Design review of the part built by this model. Coordinates are the model's own, in mm. Give positions to 0.01 mm unless a question says otherwise; leave off trailing zeros. Write each loop counter-clockwise with the first axis right and the second up, starting at its lowest first coordinate (ties: lowest second). Pieces come first, ordered by that corner, then holes. Notation, with made-up numbers: M 45.25,7 L 81.25,7 A13 cw 81.25,23 Z; hole C -15.5,-26 d5. An arc over 180 degrees is marked long. Use one line per item in the form item = value. Start each with the question number.
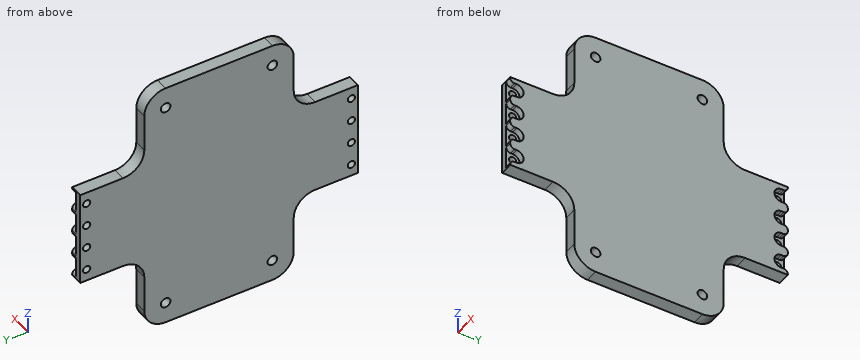
from build123d import *

# Parameters (mm, degrees)
SKETCH_1_W                  = 6
SKETCH_1_H                  = 30
EXTRUDE_1_DEPTH             = 130
EXTRUDE_3_DEPTH             = 6
HOLE_WIZARD_M31_D           = 3.4
HOLE_WIZARD_M31_CBORE_D     = 6.5
HOLE_WIZARD_M31_CBORE_DEPTH = 3
HOLE_WIZARD_M41_D           = 4.5
FILLET_1_R                  = 10
SKETCH_17_W                 = 6.5
SKETCH_17_H                 = 5
CUT_EXTRUDE_1_DEPTH         = 3
FILLET_2_R                  = 2


with BuildPart() as part:
    # Эскиз1 → Бобышка-Вытянуть1 (new body)
    with BuildSketch(Plane(origin=(0, 0, 0), x_dir=(1, 0, 0), z_dir=(0, 1, 0))):
        with Locations((3, -15)):
            Rectangle(SKETCH_1_W, SKETCH_1_H)
    extrude(amount=EXTRUDE_1_DEPTH)

    # Эскиз11 → Бобышка-Вытянуть3 (add)
    with BuildSketch(Plane(origin=(6, 0, 0), x_dir=(0, 0, -1), z_dir=(1, 0, 0))):
        Polygon((-37.5, 124), (-37.5, 100), (-75, 100), (-75, 30), (-37.5, 30), (-37.5, 6), (-37.5, 0), (7.5, 0), (7.5, 6), (7.5, 30), (45, 30), (45, 100), (7.5, 100), (7.5, 124), (7.5, 130), (-37.5, 130), align=None)
    extrude(amount=-EXTRUDE_3_DEPTH)

    # Цековка для винта с внутренним шестигранником M31 (through all)
    with Locations(Plane(origin=(6, 0, 0), x_dir=(0, 0, -1), z_dir=(1, 0, 0))):
        with Locations((-31.875, 127), (-20.625, 127), (-9.375, 127), (1.875, 127), (-31.875, 3), (-20.625, 3), (-9.375, 3), (1.875, 3)):
            CounterBoreHole(HOLE_WIZARD_M31_D / 2, HOLE_WIZARD_M31_CBORE_D / 2, HOLE_WIZARD_M31_CBORE_DEPTH)

    # Отверстие с зазором M41 (through all)
    with Locations(Plane(origin=(6, 0, 0), x_dir=(0, 0, -1), z_dir=(1, 0, 0))):
        with Locations((-65, 90), (-65, 40), (35, 40), (35, 90)):
            Hole(HOLE_WIZARD_M41_D / 2)

    # Скругление1
    fillet_1_edges = [part.edges().sort_by_distance(p)[0] for p in [
        (3, 100, -7.5),
        (3, 100, -45),
        (3, 30, -45),
        (3, 30, -7.5),
        (3, 30, 37.5),
        (3, 30, 75),
        (3, 100, 75),
        (3, 100, 37.5),
    ]]
    fillet(fillet_1_edges, radius=FILLET_1_R)

    # Эскиз17 → Вырез-Вытянуть1 (cut)
    with BuildSketch(Plane(origin=(6, 0, 0), x_dir=(0, 0, -1), z_dir=(1, 0, 0))):
        with Locations((-9.375, 129.5)):
            Rectangle(SKETCH_17_W, SKETCH_17_H)
        with Locations((1.875, 129.5)):
            Rectangle(SKETCH_17_W, SKETCH_17_H)
        with Locations((-20.625, 129.5)):
            Rectangle(SKETCH_17_W, SKETCH_17_H)
        with Locations((-31.875, 129.5)):
            Rectangle(SKETCH_17_W, SKETCH_17_H)
        with Locations((-31.875, 0.5)):
            Rectangle(SKETCH_17_W, SKETCH_17_H)
        with Locations((-20.625, 0.5)):
            Rectangle(SKETCH_17_W, SKETCH_17_H)
        with Locations((-9.375, 0.5)):
            Rectangle(SKETCH_17_W, SKETCH_17_H)
        with Locations((1.875, 0.5)):
            Rectangle(SKETCH_17_W, SKETCH_17_H)
    extrude(amount=-CUT_EXTRUDE_1_DEPTH, mode=Mode.SUBTRACT)

    # Скругление2
    fillet_2_edges = [part.edges().sort_by_distance(p)[0] for p in [
        (4.5, 130, -5.125),
        (4.5, 130, 1.375),
        (4.5, 130, 6.125),
        (4.5, 130, 12.625),
        (4.5, 130, 17.375),
        (4.5, 130, 23.875),
        (4.5, 130, 28.625),
        (4.5, 130, 35.125),
        (4.5, 0, 35.125),
        (4.5, 0, 28.625),
        (4.5, 0, 23.875),
        (4.5, 0, 17.375),
        (4.5, 0, 12.625),
        (4.5, 0, 6.125),
        (4.5, 0, 1.375),
        (4.5, 0, -5.125),
    ]]
    fillet(fillet_2_edges, radius=FILLET_2_R)


solid = part.part
1. Clearance check with flat-ended pins moving along their axes: pin 1 Ø0.5 at (x, y) = (4, 2.5) entering from +Z; pin 2 Ø4.5 at (y, z) = (3, 31.875) entering from +X; pin 3 Ø1.1 at (x, y) = (5, 2.5) entering from -Z. State where each tip first meets the part, or that it passes through.
2. To check wall thickness, follow L1, parallel to Y at x = 2.1, z = 32.5; L2, parallel to Y at x = 1.55, z = 58; L3, parallel to Y at x = 1.6, z = 30.5. State the ranges of each line that lie inside material, in increasing order.
3. We need section C-C (y = 33.5). State the section outline as (x, z) points, and give its area (3 significant figures).
4. We need section A-A (x = 4.4). Give the number of separate pieces and of enclosed holes in the cut face, and give its area (3 significant figures).
5. We need section B-B (z = 50). State the section outline as (x, y) points, and give its area (3 significant figures).
Answer block:
q1.pin_1 = 37.5
q1.pin_2 = 3
q1.pin_3 = -7.5
q2.L1 = 0 to 1.42, 4.58 to 125.42, 128.58 to 130
q2.L2 = 30 to 100
q2.L3 = 0 to 2, 4 to 126, 128 to 130
q3.outline = M 0,-42.6 L 6,-42.6 L 6,72.6 L 0,72.6 Z
q3.area = 691 mm^2
q4.separate_pieces = 1
q4.enclosed_holes = 4
q4.area = 10,700 mm^2
q5.outline = M 0,30 L 6,30 L 6,100 L 0,100 Z
q5.area = 420 mm^2
